```python
from build123d import *

# Parameters (mm, degrees)
SKETCH1_W           = 45
SKETCH1_H           = 45
SKETCH1_R           = 11
SKETCH1_R_2         = 1.5
BOSS_EXTRUDE1_DEPTH = 4
BOSS_EXTRUDE2_START = 1.649921
SKETCH2_W           = 2.999997759
SKETCH2_H           = 65
SKETCH2_W_2         = 13.199968027
SKETCH2_W_3         = 0.399954884
SKETCH2_W_4         = 11.8
SKETCH2_R           = 2
BOSS_EXTRUDE2_DEPTH = 6
BOSS_EXTRUDE4_START = -4.350079
SKETCH2_5_W         = 11.8
SKETCH2_5_H         = 65
SKETCH2_5_R         = 2
BOSS_EXTRUDE4_DEPTH = 1.5


with BuildPart() as part:
    # Sketch1 → Boss-Extrude1 (new body)
    with BuildSketch(Plane.XY):
        Rectangle(SKETCH1_W, SKETCH1_H)
        Polygon((20.15, -20.15), (20.15, -16.735786438), (20.15, 16.735786438), (16.735786438, 20.15), (-16.735786438, 20.15), (-20.15, 16.735786438), (-20.15, 16.077064234), (-20.15, -16.735786438), (-20.15, -20.15), (-16.735786438, -20.15), (16.735786438, -20.15), align=None, mode=Mode.SUBTRACT)
        Polygon((16.735786438, -20.15), (20.15, -20.15), (20.15, -16.735786438), (20.15, 16.735786438), (16.735786438, 20.15), (-16.735786438, 20.15), (-20.15, 16.735786438), (-20.15, 16.077064234), (-20.15, -16.735786438), (-20.15, -20.15), (-16.735786438, -20.15), align=None)
        Circle(SKETCH1_R, mode=Mode.SUBTRACT)
        with Locations((15.5, -15.5)):
            Circle(SKETCH1_R_2, mode=Mode.SUBTRACT)
        with Locations((15.5, 15.5)):
            Circle(SKETCH1_R_2, mode=Mode.SUBTRACT)
        with Locations((-15.5, -15.5)):
            Circle(SKETCH1_R_2, mode=Mode.SUBTRACT)
        with Locations((-15.5, 15.5)):
            Circle(SKETCH1_R_2, mode=Mode.SUBTRACT)
    extrude(amount=BOSS_EXTRUDE1_DEPTH)

    # Sketch2 → Boss-Extrude2 (add)
    with BuildSketch(Plane(origin=(0, -24.14992067, 0), x_dir=(1, 0, 0), z_dir=(0, 1, 0)).offset(BOSS_EXTRUDE2_START)):
        with Locations((21.000001121, -32.5)):
            Rectangle(SKETCH2_W, SKETCH2_H)
        with Locations((12.900018228, -32.5)):
            Rectangle(SKETCH2_W_2, SKETCH2_H)
        Polygon((-22.5, -65), (-5.89992067, -65), (-5.89992067, 0), (-19.499922911, 0), (-22.5, 0), align=None)
        with Locations((6.100056772, -32.5)):
            Rectangle(SKETCH2_W_3, SKETCH2_H)
        with Locations((7.933e-05, -32.5)):
            Rectangle(SKETCH2_W_4, SKETCH2_H)
        with Locations((-0.001608903, -59.999999943)):
            Circle(SKETCH2_R, mode=Mode.SUBTRACT)
        with Locations((7.933e-05, -35)):
            Circle(SKETCH2_R, mode=Mode.SUBTRACT)
    extrude(amount=-BOSS_EXTRUDE2_DEPTH)

    # Sketch2<5> → Boss-Extrude4 (add)
    with BuildSketch(Plane(origin=(0, -24.14992067, 0), x_dir=(1, 0, 0), z_dir=(0, 1, 0)).offset(BOSS_EXTRUDE4_START)):
        with Locations((7.933e-05, -32.5)):
            Rectangle(SKETCH2_5_W, SKETCH2_5_H)
        with Locations((-0.001608903, -59.999999943)):
            Circle(SKETCH2_5_R, mode=Mode.SUBTRACT)
        with Locations((7.933e-05, -35)):
            Circle(SKETCH2_5_R, mode=Mode.SUBTRACT)
    extrude(amount=-BOSS_EXTRUDE4_DEPTH)


solid = part.part
```
Can you work these out from the model? Positions are in its coordinate system, mm. A direction names the side the tool comes from. Give positions to 0.01 mm unless a question says otherwise; leave off trailing zeros. Order: outer loops, then holes, each group sorted by start corner. A loop starts at its lowest first (then second) coordinate and runs counter-clockwise, first axis right, second up. Notation, with made-up numbers: M 40,34.5 L 58,34.5 A27 ccw 58,58.5 Z; hole C -1,-8.5 d5. An arc over 180 degrees is marked long. Write item = value, one per line. Start each with the question number.
Q1. Will these pins go through, and if not, where does the flat tip stop? pin 1 Ø3 at (x, y) = (-7.5, -11.5) entering from -Z; pin 2 Ø5 at (x, z) = (-11, 35.5) entering from -Y; pin 3 Ø2 at (x, z) = (-2, 14) entering from +Y; pin 4 Ø0.8 at (y, z) = (-29.5, 36) entering from -X.
Q2. Suppose I cut it at A-A (x = 15.5). Write out the boundary of the cut face in (y, z), plus the area to 3 significant figures.
Q3. Suppose I cut it at C-C (y = 0). Write out the boundary of the cut face in (x, z).
Q4. We'd pull the mould along X, two halves only. Please class faces 1 (the flat face through (-22.5, -24, 20)), 2 (the cylindrical face through (14, 15.57, 1.97)), 3 (the flat face through (5, -22.5, 34)): pulls with the +X half, pulls with the -X half, needs draft (parallel to the pull), parting line crosses it, or undercut.
Q5. Suppose I cut it at D-D (z = 17). Write out the boundary of the cut face in (x, y).
Q6. For faces 4 (the flat face through (-14, -28.5, 32)), 5 (the flat face through (-5, 10, 4)), 6 (the cylindrical face through (0, -26, 37)), 7 (the flat face through (0, -25, 65)), 8 (the flat face through (14, -28.5, 32)), which set-ups out of +Z, -Z, +X, -X, +Y, -Y let a thin tool reach every point of the face, with its end or its side?
Q7. Suppose I cut it at B-B (z = 35). Write out the boundary of the cut face in (x, y), plus the area to 3 significant figures.
Q8. I need wall thicknesses on probe 1 along Y at (x, z) = (-15.5, 0.8); probe 2 along X at (y, z) = (-24.75, 35); probe 3 along Y at (x, z) = (0, 2). Which ranges of each line are inside material? Lowest first, please. Write a range as [from, to].
Check result:
q1.pin_1 = 0
q1.pin_2 = -28.5
q1.pin_3 = -22.5
q1.pin_4 = -5.9
q2.outline = M -28.5,0 L -17,0 L -17,4 L -22.5,4 L -22.5,65 L -28.5,65 Z; M -14,0 L 14,0 L 14,4 L -14,4 Z; M 17,0 L 22.5,0 L 22.5,4 L 17,4 Z
q2.area = 546 mm2
q3.outline = M -22.5,0 L -11,0 L -11,4 L -22.5,4 Z; M 11,0 L 22.5,0 L 22.5,4 L 11,4 Z
q4.face_1 = pulls with the -X half
q4.face_2 = undercut
q4.face_3 = needs draft
q5.outline = M -22.5,-28.5 L -5.9,-28.5 L -5.9,-30 L 5.9,-30 L 5.9,-28.5 L 22.5,-28.5 L 22.5,-22.5 L -22.5,-22.5 Z
q6.face_4 = +Z, -Z, -X, -Y
q6.face_5 = +Z, +X, -X, +Y
q6.face_6 = +Y, -Y
q6.face_7 = +Z, +X, -X, +Y, -Y
q6.face_8 = +Z, -Z, +X, -Y
q7.outline = M -22.5,-28.5 L -5.9,-28.5 L -5.9,-30 L -2,-30 L -2,-22.5 L -22.5,-22.5 Z; M 2,-30 L 5.9,-30 L 5.9,-28.5 L 22.5,-28.5 L 22.5,-22.5 L 2,-22.5 Z
q7.area = 258 mm2
q8.probe_1 = [-28.5, -17], [-14, 14], [17, 22.5]
q8.probe_2 = [-22.5, -2], [2, 22.5]
q8.probe_3 = [-30, -11], [11, 22.5]
